The listing builds one solid part. Answer for the finished solid, in the listing's coordinates (mm). Coordinates: 2 decimals unless noted, no trailing zeros. Write each loop counter-clockwise with the first axis right and the second up, starting at its lowest first coordinate (ties: lowest second). Pieces come first, ordered by that corner, then holes.
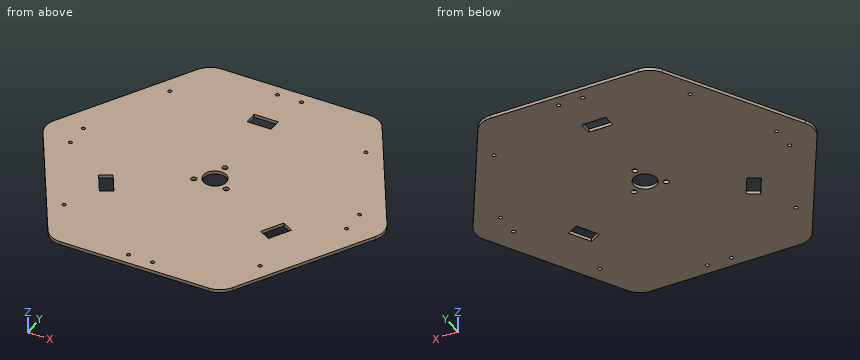
from build123d import *

# Parameters (mm, degrees)
CROQUIS1_R              = 10.8
CROQUIS1_R_2            = 2.6
CROQUIS1_W              = 22.5
CROQUIS1_H              = 12
SALIENTE_EXTRUIR1_DEPTH = 3
REDONDEO1_R             = 20
CROQUIS3_R              = 1.75
CORTAR_EXTRUIR1_DEPTH   = 212.545651301
MATRIZC1_COUNT          = 4


with BuildPart() as part:
    # Croquis1 → Saliente-Extruir1 (new body)
    with BuildSketch(Plane.XY):
        Polygon((-80.829037687, -140), (80.829037687, -140), (161.658075373, 0), (80.829037687, 140), (-80.829037687, 140), (-161.658075373, 0), align=None)
        Circle(CROQUIS1_R, mode=Mode.SUBTRACT)
        with Locations((0, 17.5)):
            Circle(CROQUIS1_R_2, mode=Mode.SUBTRACT)
        with Locations((15.155444566, -8.75)):
            Circle(CROQUIS1_R_2, mode=Mode.SUBTRACT)
        with Locations((-15.155444566, -8.75)):
            Circle(CROQUIS1_R_2, mode=Mode.SUBTRACT)
        with Locations((-3.75, 89.921841062)):
            Rectangle(CROQUIS1_W, CROQUIS1_H, mode=Mode.SUBTRACT)
        Polygon((90.570751138, -34.970539474), (80.178446292, -28.970539474), (68.928446292, -48.456111059), (79.320751138, -54.456111059), align=None, mode=Mode.SUBTRACT)
        Polygon((-75.570751138, -60.951301588), (-65.178446292, -54.951301588), (-76.428446292, -35.465730003), (-86.820751138, -41.465730003), align=None, mode=Mode.SUBTRACT)
    extrude(amount=SALIENTE_EXTRUIR1_DEPTH)

    # Redondeo1
    redondeo1_edges = [part.edges().sort_by_distance(p)[0] for p in [
        (161.658075373, 0, 1.5),
        (80.829037687, -140, 1.5),
        (-80.829037687, -140, 1.5),
        (-161.658075373, 0, 1.5),
        (-80.829037687, 140, 1.5),
        (80.829037687, 140, 1.5),
    ]]
    fillet(redondeo1_edges, radius=REDONDEO1_R)

    # Croquis3 → Cortar-Extruir1 (cut, through all)
    with BuildSketch(Plane(origin=(0, 0, 0), x_dir=(1, 0, 0), z_dir=(0, 0, -1))):
        with Locations(Location((129.505310752, 11.330246557, 0), (0, 0, 180))):
            Circle(CROQUIS3_R)
        with Locations(Location((91.923881554, 91.923881554, 0), (0, 0, 180))):
            Circle(CROQUIS3_R)
        with Locations(Location((11.330246557, 129.505310752, 0), (0, 0, 180))):
            Circle(CROQUIS3_R)
    cortar_extruir1 = extrude(amount=-CORTAR_EXTRUIR1_DEPTH, mode=Mode.SUBTRACT)

    # MatrizC1: Cortar-Extruir1 ×4 about axis
    matrizc1_axis = Axis((0, 0, 0), (0, 0, 1))
    for i in range(1, MATRIZC1_COUNT):
        add(cortar_extruir1.rotate(matrizc1_axis, i * 360 / MATRIZC1_COUNT), mode=Mode.SUBTRACT)


solid = part.part
1. Find the intervals of material crossed by L1, parallel to Y at x = 0, z = 1.7; L2, parallel to X at y = -52, z = 1.4; L3, parallel to X at y = -36, z = 1.5, in increasing order.
Results found:
L1: y = -140 to -10.8, 10.8 to 14.9, 20.1 to 83.92, 95.92 to 140
L2: x = -131.64 to -80.74, -66.88 to 75.07, 80.74 to 131.64
L3: x = -140.87 to -77.35, -76.12 to 76.12, 89.98 to 140.87
2. Section A-A on y = 0 is taken. Give the vertices of the cut face in (x, z), then the cut area to 3 significant figures.
Results found:
outline: (-158.56, 0) - (-10.8, 0) - (-10.8, 3) - (-158.56, 3) - close; (10.8, 0) - (158.56, 0) - (158.56, 3) - (10.8, 3) - close
area: 887 mm2
3. Flat-ended cylindrical pins translate along their axes: P1, Ø1.5, axis at x = -76.5, z = 0.5, coming from the -Y side; P2, Ø3, axis at x = -11.33, y = 129.51, coming from the -Z side; P3, Ø4.5, axis at x = 91.92, y = 91.92, coming from the +Z side; P4, Ø1.5, axis at y = 89, z = 2, coming from the +X side. Find the tip coordinate at first contact, or state that the pin passes through.
Results found:
P1: stops at y = -138.93
P2: passes through
P3: stops at z = 3
P4: stops at x = 110.71
4. Section D-D on x = 114 is taken. Give the vertices of the cut face in (y, z).
Results found:
outline: (-82.55, 0) - (82.55, 0) - (82.55, 3) - (-82.55, 3) - close
5. Section B-B on z = 0.9 is taken. State how many separate pieces and enclosed holes the cut face has, then the cut area to 3 significant figures.
Results found:
separate pieces: 1
enclosed holes: 19
area: 66,400 mm2
6. Section C-C on y = -117.5 is taken. Give the vertices of the cut face in (x, z).
Results found:
outline: (-93.82, 0) - (93.82, 0) - (93.82, 3) - (-93.82, 3) - close
